from build123d import *

# Parameters (mm, degrees)
BOSS_EXTRUDE1_DEPTH = 3
CUT_EXTRUDE1_REACH  = 5
SKETCH3_R           = 5.053902861
SKETCH3_R_2         = 2.749769833
BOSS_EXTRUDE2_DEPTH = 3
CUT_EXTRUDE2_REACH  = 5
SKETCH5_W           = 3
SKETCH5_H           = 8
CUT_EXTRUDE3_DEPTH  = 3


with BuildPart() as part:
    # Sketch1 → Boss-Extrude1 (new body)
    with BuildSketch(Plane.XY):
        with BuildLine():
            Line((-7, -3), (3, -3))
            Line((3, -3), (3, 0))
            Line((3, 0), (23, 0))
            Line((23, 0), (23, -3))
            Line((23, -3), (33, -3))
            Line((33, -3), (33, 0))
            Line((33, 0), (51.582575695, 0))
            ThreePointArc((51.582575695, 0), (51.894531565, 0.978451782), (52, 2))
            Line((52, 2), (52, 19.311841589))
            ThreePointArc((52, 19.311841589), (51.894531565, 20.333389808), (51.582575695, 21.311841589))
            Line((51.582575695, 21.311841589), (33, 21.311841589))
            Line((33, 21.311841589), (33, 24.311841589))
            Line((33, 24.311841589), (23, 24.311841589))
            Line((23, 24.311841589), (23, 21.311841589))
            Line((23, 21.311841589), (3, 21.311841589))
            Line((3, 21.311841589), (3, 24.311841589))
            Line((3, 24.311841589), (-7, 24.311841589))
            Line((-7, 24.311841589), (-7, 21.311841589))
            Line((-7, 21.311841589), (-25.582575695, 21.311841589))
            ThreePointArc((-25.582575695, 21.311841589), (-25.894531565, 20.333389808), (-26, 19.311841589))
            Line((-26, 19.311841589), (-26, 2))
            ThreePointArc((-26, 2), (-25.894531565, 0.978451782), (-25.582575695, 0))
            Line((-25.582575695, 0), (-7, 0))
            Line((-7, 0), (-7, -3))
        make_face()
    extrude(amount=BOSS_EXTRUDE1_DEPTH)

    # Sketch2 → Cut-Extrude1 (cut, up to next)
    with BuildSketch(Plane.XY.offset(3), mode=Mode.PRIVATE) as cut_extrude1_sk1:
        Polygon((13.38, 3.5), (13.38, 15.3), (23.54, 15.3), (52, 15.3), (52, 3.5), align=None)
    cut_extrude1_tool1 = extrude(cut_extrude1_sk1.sketch, amount=-CUT_EXTRUDE1_REACH, mode=Mode.PRIVATE) & part.part
    add(cut_extrude1_tool1.solids().sort_by_distance((32.69, 9.4, 3))[0], mode=Mode.SUBTRACT)

    # Sketch3 → Boss-Extrude2 (add)
    with BuildSketch(Plane.XY.offset(3)):
        with Locations((-20.946097139, 22.811841589)):
            Circle(SKETCH3_R)
        with Locations((-20.946097139, 22.811841589)):
            Circle(SKETCH3_R_2, mode=Mode.SUBTRACT)
    extrude(amount=-BOSS_EXTRUDE2_DEPTH)

    # Sketch4 → Cut-Extrude2 (cut, up to next)
    with BuildSketch(Plane.XY.offset(3), mode=Mode.PRIVATE) as cut_extrude2_sk1:
        with BuildLine():
            Line((-23.250708633, 21.311841589), (-18.641485645, 21.311841589))
            ThreePointArc((-18.641485645, 21.311841589), (-20.946097139, 20.062071756), (-23.250708633, 21.311841589))
        make_face()
    cut_extrude2_tool1 = extrude(cut_extrude2_sk1.sketch, amount=-CUT_EXTRUDE2_REACH, mode=Mode.PRIVATE) & part.part
    add(cut_extrude2_tool1.solids().sort_by_distance((-20.946097, 20.800705, 3))[0], mode=Mode.SUBTRACT)

    # Sketch5 → Cut-Extrude3 (cut)
    with BuildSketch(Plane.XY.offset(3)):
        with Locations((-24.5, 10.655920795)):
            Rectangle(SKETCH5_W, SKETCH5_H)
    extrude(amount=-CUT_EXTRUDE3_DEPTH, mode=Mode.SUBTRACT)


solid = part.part
CAD build for the part. Positions are in the model's coordinates, mm. A direction names the side the tool comes from. Give positions to 0.01 mm unless a question says otherwise; leave off trailing zeros. Loops run counter-clockwise (first coordinate to the right, second up) from the corner with the lowest first, then second, coordinate; pieces in that order, holes last. Notation, with made-up numbers: M -1,-37.75 L 42,-37.75 A10 ccw 42,-22.75 Z; hole C 84,-31 d8. An arc over 180 degrees is marked long. Answer in a Markdown table with one row per item. Add a question column.
Item 1: Tool access for faces 5 (the face through (23, 23, 1)), 6 (the face through (42, 0, 1)), 7 (the face through (23, -1, 1)), 8 (the face through (42, 21.312, 1)), 9 (the face through (-23, 11, 2)): list every direction of +Z, -Z, +X, -X, +Y, -Y with a clear straight run to the whole face (end or side of a thin tool).
Item 2: Band-saw the part on B-B on y = -1. Give the cut face in (x, z), then the cut area to 3 significant figures.
Item 3: Drop flat-ended pins along their axis: P1, Ø6, axis at x = 18.5, y = 2, coming from the -Z side; P2, Ø0.9, axis at y = 10.5, z = 1, coming from the +X side; P3, Ø1, axis at x = 6.5, z = 0.5, coming from the +Y side; P4, Ø1.5, axis at y = 12, z = 2, coming from the -X side. Give the stop position or say it passes through.
Item 4: Band-saw the part on D-D on y = 13. Give the cut face in (x, z), then the cut area to 3 significant figures.
Item 5: Band-saw the part on A-A on x = 40.5. Give the cut face in (y, z), then the cut area to 3 significant figures.
Item 6: Band-saw the part on C-C on y = 22.5. Give the cut face in (x, z).
Item 7: Probe probe 1 along Y at (x, z) = (37.5, 0.6); probe 2 along Y at (x, z) = (29.5, 2.1); probe 3 along Y at (x, z) = (4, 0.55). List the from-to ranges inside material, lowest first.
Item 8: Mould opens along X. For faces 1 (the face through (-25.9, 1, 1.5)), 2 (the face through (52, 3, 1)), 3 (the face through (13, 0, 1)), 4 (the face through (-2, -3, 1)) say: +X half, -X half, draft (parallel to the pull), parting line (faces both ways), or undercut.
Reply:
| question | item | result |
|---|---|---|
| 1 | face 5 | +Z, -Z, +Y |
| 1 | face 6 | +Z, -Z, +X, -Y |
| 1 | face 7 | +Z, -Z, -Y |
| 1 | face 8 | +Z, -Z, +X, +Y |
| 1 | face 9 | +Z, -Z, -X |
| 2 | outline | M -7,0 L 3,0 L 3,3 L -7,3 Z; M 23,0 L 33,0 L 33,3 L 23,3 Z |
| 2 | area | 60.0 mm^2 |
| 3 | P1 | stops at z = 0 |
| 3 | P2 | stops at x = 13.38 |
| 3 | P3 | stops at y = 21.31 |
| 3 | P4 | stops at x = -23 |
| 4 | outline | M -23,0 L 13.38,0 L 13.38,3 L -23,3 Z |
| 4 | area | 109 mm^2 |
| 5 | outline | M 0,0 L 3.5,0 L 3.5,3 L 0,3 Z; M 15.3,0 L 21.31,0 L 21.31,3 L 15.3,3 Z |
| 5 | area | 28.5 mm^2 |
| 6 | outline | M -25.99,0 L -23.68,0 L -23.68,3 L -25.99,3 Z; M -18.21,0 L -15.9,0 L -15.9,3 L -18.21,3 Z; M -7,0 L 3,0 L 3,3 L -7,3 Z; M 23,0 L 33,0 L 33,3 L 23,3 Z |
| 7 | probe 1 | y = 0 to 3.5, 15.3 to 21.31 |
| 7 | probe 2 | y = -3 to 3.5, 15.3 to 24.31 |
| 7 | probe 3 | y = 0 to 21.31 |
| 8 | face 1 | -X half |
| 8 | face 2 | +X half |
| 8 | face 3 | undercut |
| 8 | face 4 | draft |
